Geometry: final body of the model. Coordinates: model frame, mm. A direction names the side the tool comes from. Round coordinates to 2 decimals unless told otherwise and drop trailing zeros. Order: outer loops, then holes, each group sorted by start corner. A loop starts at its lowest first (then second) coordinate and runs counter-clockwise, first axis right, second up. Notation, with made-up numbers: M 27,45.5 L 66,45.5 A16 cw 66,68.5 Z; hole C 31.25,54 d10. An arc over 180 degrees is marked long. Put each result on its own line as item: value. Start each with the question number.
1) First-contact query: P1, Ø4.5, axis at y = -9.25, z = 19.92, coming from the -X side; P2, Ø5, axis at x = 8, y = -3, coming from the +Z side; P3, Ø12, axis at y = 2.5, z = 18, coming from the +X side; P4, Ø3, axis at x = -8, z = 5.5, coming from the +Y side. Flat tips, straight axial feed; report the tip coordinate or a pass-through.
2) Access query for faces 1 (the flat face through (-11, 0, 13)), 2 (the flat face through (-7, 2.54, 5)), 3 (the flat face through (-7, -2.54, 5)). Directions: +Z, -Z, +X, -X, +Y, -Y. A direction counts if a zero-diameter tool reaches every point of the face in a straight line with its end or side. Return the directions, or none.
3) Section A-A, the plane y = -9.25. Return loops of the section in (x, z).
4) Section C-C, the plane x = 7.42. Return loops of the section in (y, z).
5) Section D-D, the plane x = -4.5. Return loops of the section in (y, z).
6) Section B-B, the plane z = 19.92. Return loops of the section in (x, y).
7) Material intervals for probe 1 along Y at (x, z) = (7.42, 1.1); probe 2 along Z at (x, y) = (-11.5, -9.25); probe 3 along Z at (x, y) = (1, -5.5), sorted ascending. Write a range as [from, to].
8) Draft query along X for faces 4 (the flat face through (0, 0, 0)), 5 (the flat face through (12.5, 0, 1)), 6 (the cylindrical face through (5.436, 7.729, 0.74)). Return one class per face: pulls with the +X half, pulls with the -X half, needs draft (parallel to the pull), parting line crosses it, or undercut.
from build123d import *

# Parameters (mm, degrees)
SKETCH1_W                = 25
SKETCH1_H                = 32
SKETCH1_R                = 2.5
BOSS_EXTRUDE1_DEPTH      = 1.5
SKETCH2_W                = 25
SKETCH2_H                = 32
SKETCH2_R                = 2.5
BOSS_EXTRUDE2_DEPTH      = 1.5
BOSS_EXTRUDE3_DEPTH      = 2.54
BOSS_EXTRUDE3_DEPTH_BACK = 2.54


with BuildPart() as part:
    # Sketch1 → Boss-Extrude1 (new body)
    with BuildSketch(Plane.XY):
        Rectangle(SKETCH1_W, SKETCH1_H)
        with Locations((7.42, -9.25)):
            Circle(SKETCH1_R, mode=Mode.SUBTRACT)
        with Locations((7.42, 9.25)):
            Circle(SKETCH1_R, mode=Mode.SUBTRACT)
    extrude(amount=BOSS_EXTRUDE1_DEPTH)

    # Sketch2 → Boss-Extrude2 (add)
    with BuildSketch(Plane.ZY.offset(12.5)):
        with Locations((12.5, 0)):
            Rectangle(SKETCH2_W, SKETCH2_H)
        with Locations(Location((19.92, -9.25, 0), (0, 0, 270))):
            Circle(SKETCH2_R, mode=Mode.SUBTRACT)
        with Locations(Location((19.92, 9.25, 0), (0, 0, 270))):
            Circle(SKETCH2_R, mode=Mode.SUBTRACT)
    extrude(amount=-BOSS_EXTRUDE2_DEPTH)

    # Sketch3 → Boss-Extrude3 (add, two sides: drawn at the far end of the back side and taken through both)
    with BuildSketch(Plane(origin=(0, 0, 0), x_dir=(1, 0, 0), z_dir=(0, 1, 0)).offset(-BOSS_EXTRUDE3_DEPTH_BACK)):
        Polygon((-11, -1.5), (-11, -11.66), (-0.84, -1.5), align=None)
    extrude(amount=BOSS_EXTRUDE3_DEPTH + BOSS_EXTRUDE3_DEPTH_BACK)


solid = part.part
Result sheet:
1. P1: passes through
1. P2: stops at z = 1.5
1. P3: stops at x = -11
1. P4: stops at y = 2.54
2. face 1: +Z, +X
2. face 2: +Z, +X, +Y
2. face 3: +Z, +X, -Y
3. outline: M -12.5,0 L 4.92,0 L 4.92,1.5 L -11,1.5 L -11,17.42 L -12.5,17.42 Z; M -12.5,22.42 L -11,22.42 L -11,25 L -12.5,25 Z; M 9.92,0 L 12.5,0 L 12.5,1.5 L 9.92,1.5 Z
4. outline: M -16,0 L -11.75,0 L -11.75,1.5 L -16,1.5 Z; M -6.75,0 L 6.75,0 L 6.75,1.5 L -6.75,1.5 Z; M 11.75,0 L 16,0 L 16,1.5 L 11.75,1.5 Z
5. outline: M -16,0 L 16,0 L 16,1.5 L 2.54,1.5 L 2.54,5.16 L -2.54,5.16 L -2.54,1.5 L -16,1.5 Z
6. outline: M -12.5,-16 L -11,-16 L -11,-11.75 L -12.5,-11.75 Z; M -12.5,-6.75 L -11,-6.75 L -11,6.75 L -12.5,6.75 Z; M -12.5,11.75 L -11,11.75 L -11,16 L -12.5,16 Z
7. probe 1: y = [-16, -11.75], [-6.75, 6.75], [11.75, 16]
7. probe 2: z = [0, 17.42], [22.42, 25]
7. probe 3: z = [0, 1.5]
8. face 4: needs draft
8. face 5: pulls with the +X half
8. face 6: undercut
